```python
from build123d import *

# Parameters (mm, degrees)
SKETCH2_W           = 42
SKETCH2_H           = 80
BOSS_EXTRUDE1_DEPTH = 46
SKETCH3_W           = 66
SKETCH3_H           = 23
BOSS_EXTRUDE2_DEPTH = 19
SKETCH4_R           = 5
BOSS_EXTRUDE3_DEPTH = 4
SKETCH5_R           = 33.5
BOSS_EXTRUDE4_DEPTH = 25
SKETCH6_W           = 66
SKETCH6_H           = 23
BOSS_EXTRUDE5_DEPTH = 19
BOSS_EXTRUDE6_START = 4
SKETCH8_R           = 5
BOSS_EXTRUDE6_DEPTH = 4
SKETCH10_R          = 33
BOSS_EXTRUDE7_DEPTH = 25
FILLET2_R           = 3


with BuildPart() as part:
    # Sketch2 → Boss-Extrude1 (new body)
    with BuildSketch(Plane(origin=(0, 0, 0), x_dir=(1, 0, 0), z_dir=(0, 1, 0))):
        with Locations((55.96969697, 0.151515152)):
            Rectangle(SKETCH2_W, SKETCH2_H)
    extrude(amount=BOSS_EXTRUDE1_DEPTH)

    # Sketch3 → Boss-Extrude2 (add)
    with BuildSketch(Plane(origin=(76.96969697, 0, 0), x_dir=(0, 0, -1), z_dir=(1, 0, 0))):
        with Locations((-6.848484848, 11.5)):
            Rectangle(SKETCH3_W, SKETCH3_H)
    extrude(amount=BOSS_EXTRUDE2_DEPTH)

    # Sketch4 → Boss-Extrude3 (add)
    with BuildSketch(Plane(origin=(95.96969697, 0, 0), x_dir=(0, 0, -1), z_dir=(1, 0, 0))):
        with Locations(Location((-29.848484848, 11.5, 0), (0, 0, 180))):
            Circle(SKETCH4_R)
    extrude(amount=BOSS_EXTRUDE3_DEPTH)

    # Sketch5 → Boss-Extrude4 (add)
    with BuildSketch(Plane(origin=(99.96969697, 0, 0), x_dir=(0, 0, -1), z_dir=(1, 0, 0))):
        with Locations((-29.848484848, 11.5)):
            Circle(SKETCH5_R)
    extrude(amount=BOSS_EXTRUDE4_DEPTH)

    # Sketch6 → Boss-Extrude5 (add)
    with BuildSketch(Plane.ZY.offset(-34.96969697)):
        with Locations((6.848484848, 11.5)):
            Rectangle(SKETCH6_W, SKETCH6_H)
    extrude(amount=BOSS_EXTRUDE5_DEPTH)

    # Sketch8 → Boss-Extrude6 (add)
    with BuildSketch(Plane.ZY.offset(-15.96969697).offset(BOSS_EXTRUDE6_START)):
        with Locations((29.848484848, 11.5)):
            Circle(SKETCH8_R)
    extrude(amount=-BOSS_EXTRUDE6_DEPTH)

    # Sketch10 → Boss-Extrude7 (add)
    with BuildSketch(Plane.ZY.offset(-11.96969697)):
        with Locations((29.848484848, 11.5)):
            Circle(SKETCH10_R)
    extrude(amount=BOSS_EXTRUDE7_DEPTH)

    # Fillet2
    fillet2_edges = [part.edges().sort_by_distance(p)[0] for p in [
        (99.96969697, 11.5, 63.348484848),
        (124.96969697, 11.5, 63.348484848),
        (11.96969697, 11.5, -3.151515152),
        (-13.03030303, 11.5, -3.151515152),
    ]]
    fillet(fillet2_edges, radius=FILLET2_R)


solid = part.part
```
CAD build for the part. Positions are in the model's coordinates, mm. A direction names the side the tool comes from. Coordinates: 2 decimals unless noted, no trailing zeros. Write each loop counter-clockwise with the first axis right and the second up, starting at its lowest first coordinate (ties: lowest second). Pieces come first, ordered by that corner, then holes.
(1) Flat gauge pins, fed straight in: pin 1 (4 mm diameter, centred on y = 13, z = -29.5, fed in from -X); pin 2 (5.5 mm diameter, centred on x = 30, z = 11, fed in from +Y); pin 3 (3 mm diameter, centred on x = 74.5, y = 26, fed in from +Z); pin 4 (3 mm diameter, centred on x = 51.5, z = 40, fed in from +Y). Where does each tip first touch, or does it go through?
(2) Two-plate mould, pull along X, no slides. Class faces 4 (the face through (-13.03, 12, 29)), 5 (the face through (56, 46, -1)), 6 (the face through (57, 0, -1)), 7 (the face through (86, 23, 7)): +X half, -X half, draft (parallel to the pull), parting line (faces both ways), or undercut.
(3) Drill centre lines: probe 1 along X at (y, z) = (22.5, 23); probe 2 along X at (y, z) = (-5, 38); probe 3 along Y at (x, z) = (74.5, -33). Where is each one in solid material? Low to high.
(4) Cut at C-C, the plane x = 21. List the corners of the cut face in (y, z), and give its area (3 significant figures).
(5) Cut at D-D, the plane z = 12. Count the separate pieces of the cut face and the enclosed holes in it, and give its area (3 significant figures).
(6) Cut at A-A, the plane z = -24. List the corners of the cut face in (x, y), and give its area (3 significant figures).
(7) 3-axis set-ups, long thin cutter, end or side, ignore diameter. For faces 1 (the face through (86, 11, -26.152)), 2 (the face through (112.337, 21.562, -2.105)), 3 (the face through (97.942, 7.284, 32.536)): which of +Z, -Z, +X, -X, +Y, -Y reach the whole face in a straight line?
Geometry says:
1. pin 1: stops at x = 34.97
1. pin 2: stops at y = 23
1. pin 3: stops at z = 39.85
1. pin 4: stops at y = 46
2. face 4: -X half
2. face 5: draft
2. face 6: undercut
2. face 7: undercut
3. probe 1: x = -13.03 to 11.97, 15.97 to 95.97, 99.97 to 124.97
3. probe 2: x = -13.03 to 11.97, 99.97 to 124.97
3. probe 3: y = 0 to 46
4. outline: (0, -26.15) - (23, -26.15) - (23, 39.85) - (0, 39.85) - close
4. area: 1,520 mm2
5. separate pieces: 3
5. enclosed holes: 0
5. area: 5,590 mm2
6. outline: (15.97, 0) - (95.97, 0) - (95.97, 23) - (76.97, 23) - (76.97, 46) - (34.97, 46) - (34.97, 23) - (15.97, 23) - close
6. area: 2,810 mm2
7. face 1: -Z, +X, +Y, -Y
7. face 2: +X
7. face 3: none
